Geometry: see drawing. Coordinates: mm, zero at the bounding-box minimum. A direction names the side the tool comes from. Coordinates: 2 decimals unless noted, no trailing zeros. Write each loop counter-clockwise with the first axis right and the second up, starting at its lowest first coordinate (ties: lowest second). Pieces come first, ordered by that corner, then holes. Notation, with made-up numbers: (-27, -29) - (0, -29) arc R23 cw to (0, 9) - close; hole circle Ø1 at (-15, 9.25). An arc over 180 degrees is marked (long way). Use a Markdown table: item, result. Add a question column.
Q1. Pin query (flat end, axial travel): P1, Ø0.7, axis at x = 2.5, y = 1.5, coming from the -Z side; P2, Ø0.5, axis at x = 4, z = 2.5, coming from the +Y side; P3, Ø0.9, axis at x = 2, z = 9.5, coming from the -Y side. Return the tip coordinate at first contact, or that it passes through.
Q2. Mould query, pull axis Z, two halves, no side actions, for the marked faces 1 and 2. Classes: released by +Z, released by -Z, zero draft, split by the parting line, or undercut.
Q3. Material intervals for probe 1 along X at (y, z) = (1.55, 4.5); probe 2 along Z at (x, y) = (2.5, 1.3); probe 3 along X at (y, z) = (1.45, 12.25), sorted ascending. Write a range as from..to.
Q4. Section query D-D (x = 7.5). Return the cut outline in (y, z).
Q5. Section query C-C (x = 2.75). Return the cut outline in (y, z).
Q6. Set-up query: the marked faces 3 and 4. Return all of +Z, -Z, +X, -X, +Y, -Y with unobstructed straight access to the full face (end or side cutting, diameter ignored); none if empty.
Q7. Section query A-A (z = 9). Return the cut outline in (x, y).
Q8. Section query B-B (x = 4). Return the cut outline in (y, z).
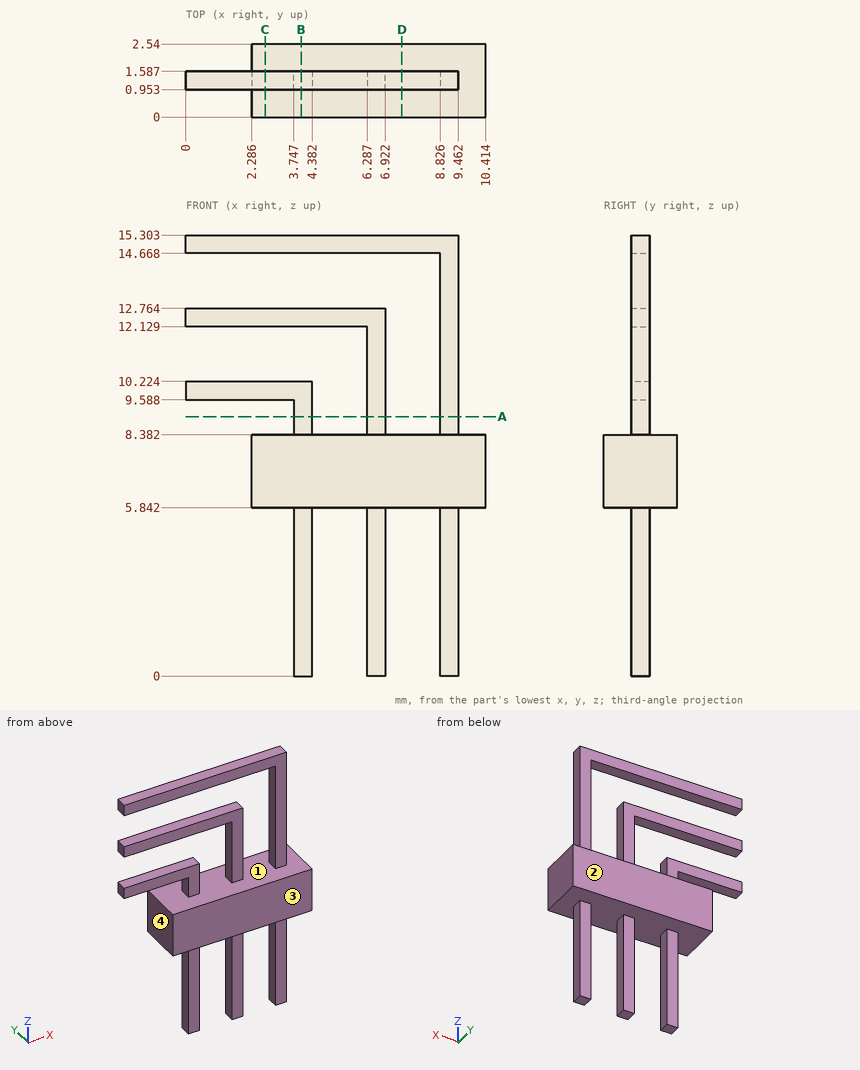
Values follow:
| question | item | result |
|---|---|---|
| 1 | P1 | z = 5.84 |
| 1 | P2 | y = 1.59 |
| 1 | P3 | y = 0.95 |
| 2 | face 1 | undercut |
| 2 | face 2 | zero draft |
| 3 | probe 1 | 3.75..4.38, 6.29..6.92, 8.83..9.46 |
| 3 | probe 2 | 5.84..8.38, 9.59..10.22, 12.13..12.76, 14.67..15.3 |
| 3 | probe 3 | 0..6.92, 8.83..9.46 |
| 4 | outline | (0, 5.84) - (2.54, 5.84) - (2.54, 8.38) - (0, 8.38) - close; (0.95, 14.67) - (1.59, 14.67) - (1.59, 15.3) - (0.95, 15.3) - close |
| 5 | outline | (0, 5.84) - (2.54, 5.84) - (2.54, 8.38) - (0, 8.38) - close; (0.95, 9.59) - (1.59, 9.59) - (1.59, 10.22) - (0.95, 10.22) - close; (0.95, 12.13) - (1.59, 12.13) - (1.59, 12.76) - (0.95, 12.76) - close; (0.95, 14.67) - (1.59, 14.67) - (1.59, 15.3) - (0.95, 15.3) - close |
| 6 | face 3 | +Z, -Z, +X, -X, -Y |
| 6 | face 4 | -Z, -X, +Y, -Y |
| 7 | outline | (3.75, 0.95) - (4.38, 0.95) - (4.38, 1.59) - (3.75, 1.59) - close; (6.29, 0.95) - (6.92, 0.95) - (6.92, 1.59) - (6.29, 1.59) - close; (8.83, 0.95) - (9.46, 0.95) - (9.46, 1.59) - (8.83, 1.59) - close |
| 8 | outline | (0, 5.84) - (0.95, 5.84) - (0.95, 0) - (1.59, 0) - (1.59, 5.84) - (2.54, 5.84) - (2.54, 8.38) - (1.59, 8.38) - (1.59, 10.22) - (0.95, 10.22) - (0.95, 8.38) - (0, 8.38) - close; (0.95, 12.13) - (1.59, 12.13) - (1.59, 12.76) - (0.95, 12.76) - close; (0.95, 14.67) - (1.59, 14.67) - (1.59, 15.3) - (0.95, 15.3) - close |
